```python
from build123d import *

# Parameters (mm, degrees)
F0_R          = 6
F1_DEPTH      = 50
F1_DEPTH_BACK = 50
F2_R          = 8
F2_R_2        = 6
F4_DEPTH      = 25
F3_R          = 8
F3_R_2        = 6
F5_DEPTH      = 25
F6_S5_R       = 6
F6_T6_DEPTH   = 14
F6_S11_R      = 6
F6_T12_DEPTH  = 14
F7_R          = 6.1
F8_DEPTH      = 9
F9_R          = 6.1
F10_DEPTH     = 9


# Not quite as in the source:
# - a fillet or chamfer that OpenCascade refuses, or shapes differently, is made with other operations: its cross-section is extruded or revolved along the edge and cut away or added


with BuildPart() as f1:
    # F0 (on Top) → F1 (new body, two sides)
    with BuildSketch(Plane.XY) as f1_sk:
        Circle(F0_R)
    extrude(amount=F1_DEPTH)
    extrude(f1_sk.sketch, amount=-F1_DEPTH_BACK)

    # F2 (on face) → F4 (join)
    with BuildSketch(Plane.XY.offset(50)):
        Circle(F2_R)
        Circle(F2_R_2, mode=Mode.SUBTRACT)
        Circle(F2_R_2)
    extrude(amount=F4_DEPTH)

    # F3 (on face) → F5 (join)
    with BuildSketch(Plane(origin=(0, 0, -50), x_dir=(1, 0, 0), z_dir=(0, 0, -1))):
        Circle(F3_R)
        Circle(F3_R_2, mode=Mode.SUBTRACT)
        Circle(F3_R_2)
    extrude(amount=F5_DEPTH)

    # F6: chamfer of 8 x 2.1435935394 on 2 edges, made by hand


with BuildPart() as f6_tool2:
    # F6_s3 → F6_t4 (revolve)
    with BuildSketch(Plane.XZ):
        Polygon((8, -58), (5.8564064606, -50), (8, -50), align=None)
    revolve(axis=Axis((0, 0, -50), (0, 0, -1)))

    # F6_s5 → F6_t6 (cut, symmetric)
    with BuildSketch(Plane.XY.offset(-54)):
        Circle(F6_S5_R)
    extrude(amount=F6_T6_DEPTH, both=True, mode=Mode.SUBTRACT)


with BuildPart() as f1_1:
    add(f1.part)

    # F6_t1: cut F6_tool2
    add(f6_tool2.part, mode=Mode.SUBTRACT)


with BuildPart() as f6_tool8:
    # F6_s9 → F6_t10 (revolve)
    with BuildSketch(Plane.XZ):
        Polygon((5.8564064606, 50), (8, 58), (8, 50), align=None)
    revolve(axis=Axis((0, 0, 50), (0, 0, 1)))

    # F6_s11 → F6_t12 (cut, symmetric)
    with BuildSketch(Plane.XY.offset(54)):
        Circle(F6_S11_R)
    extrude(amount=F6_T12_DEPTH, both=True, mode=Mode.SUBTRACT)


with BuildPart() as f1_2:
    add(f1_1.part)

    # F6_t7: cut F6_tool8
    add(f6_tool8.part, mode=Mode.SUBTRACT)

    # F7 (on face) → F8 (cut)
    with BuildSketch(Plane(origin=(0, 0, -75), x_dir=(1, 0, 0), z_dir=(0, 0, -1))):
        Circle(F7_R)
    extrude(amount=-F8_DEPTH, mode=Mode.SUBTRACT)

    # F9 (on face) → F10 (cut)
    with BuildSketch(Plane.XY.offset(75)):
        Circle(F9_R)
    extrude(amount=-F10_DEPTH, mode=Mode.SUBTRACT)


solid = f1_2.part
```
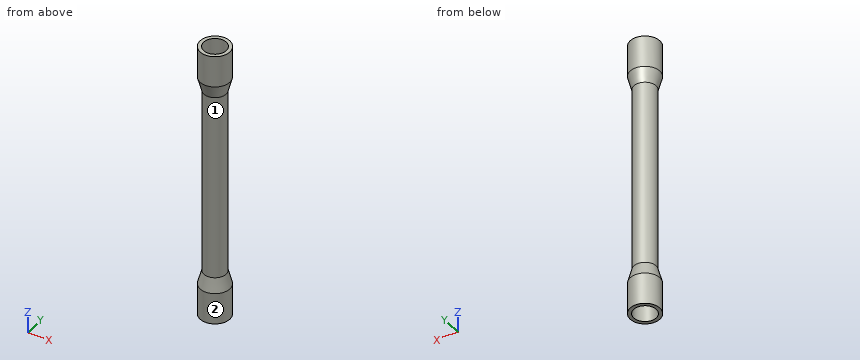
Part model, mm, in its own coordinate system. Face numbers are marked on the shaded views. A direction names the side the tool comes from. Coordinates: 2 decimals unless noted, no trailing zeros. Order: outer loops, then holes, each group sorted by start corner. A loop starts at its lowest first (then second) coordinate and runs counter-clockwise, first axis right, second up. Notation, with made-up numbers: (52, 49) - (81, 49) arc R29 cw to (81, 69) - close; hole circle Ø2 at (3.5, 1.25). An arc over 180 degrees is marked (long way). Return JSON: item names as keys, results as strings. Group by question number.
Item 1: Drill centre lines: probe 1 along X at (y, z) = (0, -72); probe 2 along Y at (x, z) = (0.5, -62). Where is each one in solid material? Low to high. Write a range as from..to.
Item 2: Cut at A-A (x = 0). List the corners of the cut face in (y, z), plus the area to 3 significant figures.
Item 3: Cut at C-C (z = -41). List the corners of the cut face in (x, y), plus the area to 3 significant figures.
Item 4: Which spindle directions (+Z, -Z, +X, -X, +Y, -Y) get a long thin tool onto all of the face, cutting with end or side? Do the marked faces 1 and 2. Say none if no direction does.
Item 5: Pin check, flat tips, straight feed: pin 1 (3.5 mm diameter, centred on x = -1, y = 1, fed in from +Z); pin 2 (2 mm diameter, centred on y = -3.5, z = 25.5, fed in from +X); pin 3 (6 mm diameter, centred on x = -3, z = -36, fed in from -Y). Stop position of each tip, or through.
Check values:
{
 "1": {"probe 1": "x = -8..-6.1, 6.1..8", "probe 2": "y = -7.98..7.98"},
 "2": {"outline": "(-8, -75) - (-6.1, -75) - (-6.1, -66) - (6.1, -66) - (6.1, -75) - (8, -75) - (8, -58) - (6, -50.54) - (6, 50.54) - (8, 58) - (8, 75) - (6.1, 75) - (6.1, 66) - (-6.1, 66) - (-6.1, 75) - (-8, 75) - (-8, 58) - (-6, 50.54) - (-6, -50.54) - (-8, -58) - close", "area": "1,750 mm2"},
 "3": {"outline": "circle Ø12 at (0, 0)", "area": "113 mm2"},
 "4": {"face 1": "none", "face 2": "+Z, -Z"},
 "5": {"pin 1": "stops at z = 66", "pin 2": "stops at x = 5.45", "pin 3": "stops at y = -6"}
}
